Geometry check sheet. Reference: the model listing, model coordinates, mm. Face numbers are marked on the shaded views. A direction names the side the tool comes from. Give positions to 0.01 mm unless a question says otherwise; leave off trailing zeros. Loops run counter-clockwise (first coordinate to the right, second up) from the corner with the lowest first, then second, coordinate; pieces in that order, holes last. Notation, with made-up numbers: (-24.5, 85) - (-11.5, 85) arc R28 cw to (-11.5, 122) - close; hole circle Ø10 at (2.5, -12.5). An arc over 180 degrees is marked (long way). Use a Markdown table: item, result. Add a question column.
1. Material ranges on L1, parallel to Z at x = -36.5, y = 54.95; L2, parallel to X at y = 52, z = -15; L3, parallel to Y at x = -0.5, z = -17, recorded low to high.
2. Draft check along Y on the marked faces 1, 2 and 3. Enter one of: pulls with the +Y half, pulls with the -Y half, needs draft (parallel to the pull), parting line crosses it, or undercut.
3. Cross-section at D-D on x = -18. Enter the section's corners in (y, z), and give its area (3 significant figures).
4. Set-up check for the marked faces 4, 5 and 6: record each of +Z, -Z, +X, -X, +Y, -Y from which the full face is reachable in a straight line by a thin tool's end or side.
5. Cross-section at A-A on z = 15. Enter the section's corners in (x, y), and give its area (4 significant figures).
6. Cross-section at B-B on y = -10. Enter the section's corners in (x, z).
7. Depth check by flat-ended pin: P1, Ø3.5, axis at x = -5.5, z = -15, coming from the -Y side; P2, Ø8, axis at x = -1, z = 5, coming from the +Y side; P3, Ø12, axis at y = 45, z = -0.5, coming from the -X side; P4, Ø1.8, axis at x = -36.5, z = -15, coming from the +Y side. Enter the tip coordinate at first touch or a pass-through.
8. Cross-section at C-C on x = -5.5. Enter the section's corners in (y, z), and give its area (3 significant figures).
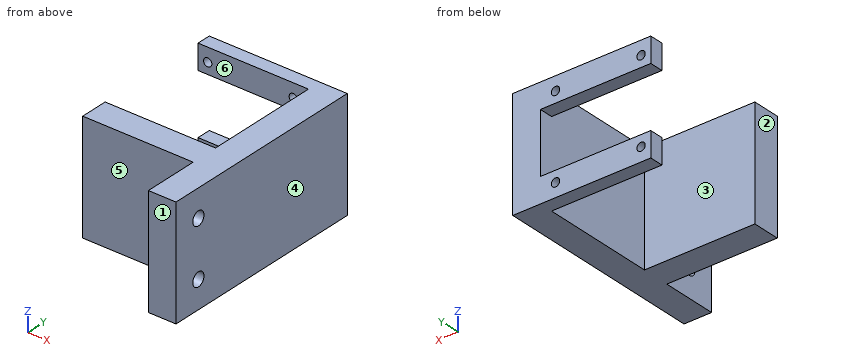
from build123d import *

# Parameters (mm, degrees)
SKETCH1_W           = 40
SKETCH1_H           = 56.5
SKETCH1_H_2         = 20
SKETCH1_R           = 2.5
BOSS_EXTRUDE1_DEPTH = 10
SKETCH3_W           = 40
SKETCH3_H           = 10
BOSS_EXTRUDE2_DEPTH = 40
SKETCH4_W           = 9
SKETCH4_H           = 5
BOSS_EXTRUDE3_DEPTH = 40
SKETCH5_R           = 1.5
CUT_EXTRUDE1_DEPTH  = 5


with BuildPart() as part:
    # Sketch1 → Boss-Extrude1 (new body)
    with BuildSketch(Plane(origin=(0, 0, 0), x_dir=(0, 0, -1), z_dir=(1, 0, 0))):
        with Locations((0, 28.25)):
            Rectangle(SKETCH1_W, SKETCH1_H)
        with Locations((0, -10)):
            Rectangle(SKETCH1_W, SKETCH1_H_2)
        with Locations((10, -10)):
            Circle(SKETCH1_R, mode=Mode.SUBTRACT)
        with Locations((-10, -10)):
            Circle(SKETCH1_R, mode=Mode.SUBTRACT)
    extrude(amount=BOSS_EXTRUDE1_DEPTH)

    # Sketch3 → Boss-Extrude2 (add)
    with BuildSketch(Plane.ZY):
        with Locations((0, 5)):
            Rectangle(SKETCH3_W, SKETCH3_H)
    extrude(amount=BOSS_EXTRUDE2_DEPTH)

    # Sketch4 → Boss-Extrude3 (add)
    with BuildSketch(Plane.ZY):
        with Locations((-15.5, 54)):
            Rectangle(SKETCH4_W, SKETCH4_H)
    boss_extrude3 = extrude(amount=BOSS_EXTRUDE3_DEPTH)

    # Sketch5 → Cut-Extrude1 (cut)
    with BuildSketch(Plane(origin=(0, 56.5, 0), x_dir=(1, 0, 0), z_dir=(0, 1, 0))):
        with Locations((-36.5, 15)):
            Circle(SKETCH5_R)
        with Locations((-5.5, 15)):
            Circle(SKETCH5_R)
    cut_extrude1 = extrude(amount=-CUT_EXTRUDE1_DEPTH, mode=Mode.SUBTRACT)

    # Mirror2: Boss-Extrude3, Cut-Extrude1 across plane
    add(boss_extrude3.mirror(Plane.XY))
    add(cut_extrude1.mirror(Plane.XY), mode=Mode.SUBTRACT)


solid = part.part
Values found:
| question | item | result |
|---|---|---|
| 1 | L1 | z = -20 to -16.5, -13.5 to -11, 11 to 13.5, 16.5 to 20 |
| 1 | L2 | x = -40 to -38, -35 to -7, -4 to 10 |
| 1 | L3 | y = 0 to 10, 51.5 to 56.5 |
| 2 | face 1 | pulls with the -Y half |
| 2 | face 2 | needs draft |
| 2 | face 3 | undercut |
| 3 | outline | (0, -20) - (10, -20) - (10, 20) - (0, 20) - close; (51.5, -20) - (56.5, -20) - (56.5, -11) - (51.5, -11) - close; (51.5, 11) - (56.5, 11) - (56.5, 20) - (51.5, 20) - close |
| 3 | area | 490 mm2 |
| 4 | face 4 | +Z, -Z, +X, +Y, -Y |
| 4 | face 5 | +Z, -Z, -X, -Y |
| 4 | face 6 | +Z, -Z, -X |
| 5 | outline | (-40, 0) - (0, 0) - (0, -20) - (10, -20) - (10, 56.5) - (-4, 56.5) - (-4, 51.5) - (0, 51.5) - (0, 10) - (-40, 10) - close; (-40, 51.5) - (-38, 51.5) - (-38, 56.5) - (-40, 56.5) - close; (-35, 51.5) - (-7, 51.5) - (-7, 56.5) - (-35, 56.5) - close |
| 5 | area | 1,335 mm2 |
| 6 | outline | (0, -20) - (10, -20) - (10, -12.5) - (0, -12.5) - close; (0, -7.5) - (10, -7.5) - (10, 7.5) - (0, 7.5) - close; (0, 12.5) - (10, 12.5) - (10, 20) - (0, 20) - close |
| 7 | P1 | stops at y = 0 |
| 7 | P2 | stops at y = 56.5 |
| 7 | P3 | stops at x = 0 |
| 7 | P4 | stops at y = 10 |
| 8 | outline | (0, -20) - (10, -20) - (10, 20) - (0, 20) - close; (51.5, -20) - (56.5, -20) - (56.5, -16.5) - (51.5, -16.5) - close; (51.5, -13.5) - (56.5, -13.5) - (56.5, -11) - (51.5, -11) - close; (51.5, 11) - (56.5, 11) - (56.5, 13.5) - (51.5, 13.5) - close; (51.5, 16.5) - (56.5, 16.5) - (56.5, 20) - (51.5, 20) - close |
| 8 | area | 460 mm2 |
